For this review, use the dimensioned drawing (mm, ordinates from the lowest corner) and the shaded views. A direction names the side the tool comes from. Coordinates: 2 decimals unless noted, no trailing zeros. Loops run counter-clockwise (first coordinate to the right, second up) from the corner with the lowest first, then second, coordinate; pieces in that order, holes last. Notation, with made-up numbers: M 4,60 L 14,60 A7 cw 14,65 Z; hole C 77.5,-16 d9. An arc over 180 degrees is marked long. Write item = value, one per line.
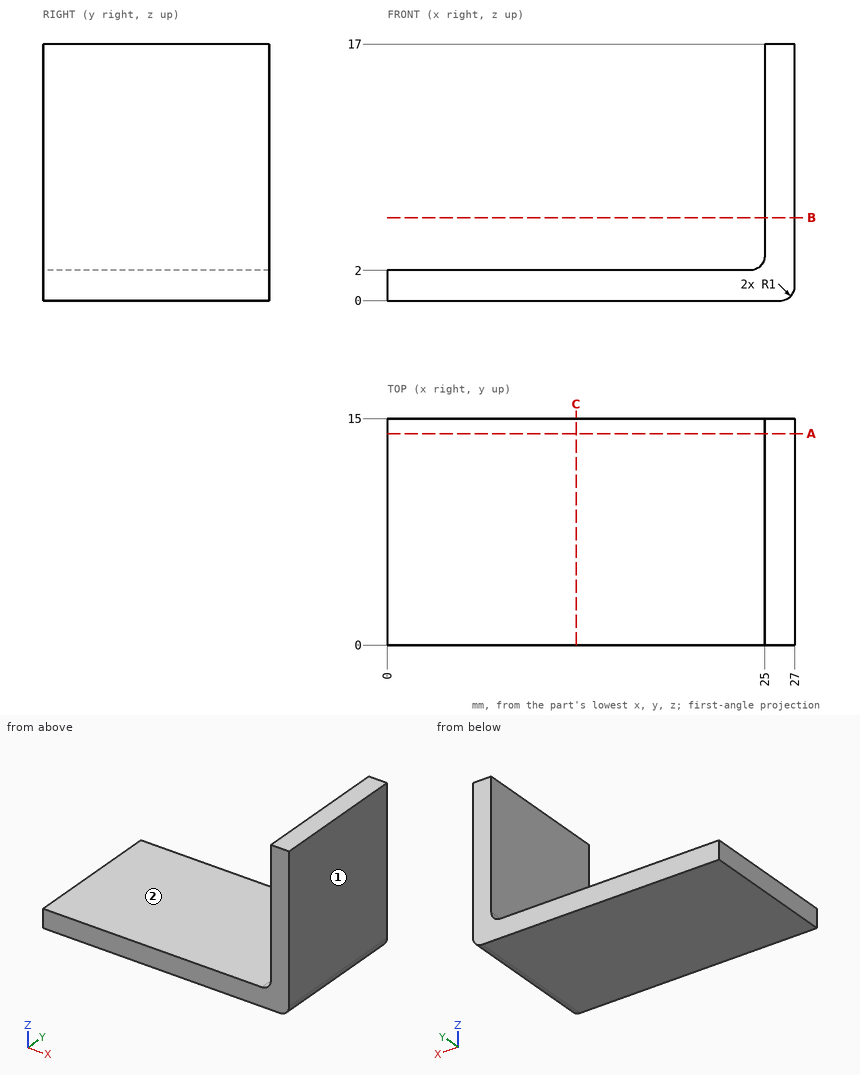
Q1. Add section B-B (z = 5.5). Write out the cut boundary in (x, y).
Solved:
outline = M 25,0 L 27,0 L 27,15 L 25,15 Z
Q2. Add section A-A (y = 14). Write out the cut boundary in (x, z).
Solved:
outline = M 0,0 L 26,0 A1 ccw 27,1 L 27,17 L 25,17 L 25,3 A1 cw 24,2 L 0,2 Z
Q3. For pin 1 Ø4 at (x, y) = (6, 2.5) entering from +Z; pin 2 Ø7 at (y, z) = (10.5, 12.5) entering from -X, all flat-tipped, find the tip position at first contact; note any pin that passes through.
Solved:
pin_1 = 2
pin_2 = 25
Q4. Add section C-C (x = 12.5). Write out the cut boundary in (y, z).
Solved:
outline = M 0,0 L 15,0 L 15,2 L 0,2 Z
Q5. For line 1 along X through (y, z) = (13.25, 13.5); line 2 along Z through (x, y) = (22, 8.75), list the stretches that pass through material, from the lowest coordinate up.
Solved:
line_1 = 25 to 27
line_2 = 0 to 2
Q6. Machinability: for the marked faces 1 and 2, which of the approach directions +Z, -Z, +X, -X, +Y, -Y give a long, thin tool a straight path to every point of the face, cutting with its end or side? Answer none if there is none.
Solved:
face_1 = +Z, -Z, +X, +Y, -Y
face_2 = +Z, -X, +Y, -Y
